```python
from build123d import *

# Parameters (mm, degrees)
SKETCH1_W           = 369
SKETCH1_H           = 81
BOSS_EXTRUDE1_DEPTH = 10
SKETCH2_W           = 23
SKETCH2_H           = 162
BOSS_EXTRUDE2_DEPTH = 38
SKETCH3_R           = 3.3
CUT_EXTRUDE1_DEPTH  = 13
SKETCH4_R           = 2.5
CUT_EXTRUDE2_DEPTH  = 163
SKETCH5_R           = 1.65
CUT_EXTRUDE3_DEPTH  = 24
CUT_EXTRUDE4_DEPTH  = 13


with BuildPart() as part:
    # Sketch1 → Boss-Extrude1 (new body)
    with BuildSketch(Plane.XY):
        with Locations((184.5, 40.5)):
            Rectangle(SKETCH1_W, SKETCH1_H)
    extrude(amount=BOSS_EXTRUDE1_DEPTH)

    # Sketch2 → Boss-Extrude2 (add)
    with BuildSketch(Plane(origin=(369, 0, 0), x_dir=(0, 0, -1), z_dir=(1, 0, 0))):
        with Locations((-11.5, 0)):
            Rectangle(SKETCH2_W, SKETCH2_H)
    extrude(amount=BOSS_EXTRUDE2_DEPTH)

    # Sketch3 → Cut-Extrude1 (cut)
    with BuildSketch(Plane(origin=(0, 0, 0), x_dir=(-1, 0, 0), z_dir=(0, 0, -1))):
        with Locations((-10, 71)):
            Circle(SKETCH3_R)
        with Locations((-10, 10)):
            Circle(SKETCH3_R)
        with Locations((-40, 10)):
            Circle(SKETCH3_R)
        with Locations((-40, 71)):
            Circle(SKETCH3_R)
    extrude(amount=-CUT_EXTRUDE1_DEPTH, mode=Mode.SUBTRACT)

    # Sketch4 → Cut-Extrude2 (cut, through all)
    with BuildSketch(Plane(origin=(0, 81, 0), x_dir=(1, 0, 0), z_dir=(0, 1, 0))):
        with Locations((388, -11.5)):
            Circle(SKETCH4_R)
    extrude(amount=-CUT_EXTRUDE2_DEPTH, mode=Mode.SUBTRACT)

    # Sketch5 → Cut-Extrude3 (cut, through all)
    with BuildSketch(Plane(origin=(0, 0, 0), x_dir=(-1, 0, 0), z_dir=(0, 0, -1))):
        with Locations((-378, -78)):
            Circle(SKETCH5_R)
        with Locations((-378, 78)):
            Circle(SKETCH5_R)
    extrude(amount=-CUT_EXTRUDE3_DEPTH, mode=Mode.SUBTRACT)

    # Sketch6 → Cut-Extrude4 (cut)
    with BuildSketch(Plane(origin=(0, 0, 0), x_dir=(-1, 0, 0), z_dir=(0, 0, -1))):
        with BuildLine():
            Line((-382, -78), (-382, -81))
            Line((-382, -81), (-374, -81))
            Line((-374, -81), (-374, -78))
            ThreePointArc((-374, -78), (-378, -74), (-382, -78))
        make_face()
        with BuildLine():
            Line((-374, 78), (-374, 81))
            Line((-374, 81), (-382, 81))
            Line((-382, 81), (-382, 78))
            ThreePointArc((-382, 78), (-378, 74), (-374, 78))
        make_face()
    extrude(amount=-CUT_EXTRUDE4_DEPTH, mode=Mode.SUBTRACT)


solid = part.part
```
Input: part model. Units: mm. Frame: model coordinates. A direction names the side the tool comes from. Round coordinates to 2 decimals unless told otherwise and drop trailing zeros. Write each loop counter-clockwise with the first axis right and the second up, starting at its lowest first coordinate (ties: lowest second). Pieces come first, ordered by that corner, then holes. Notation, with made-up numbers: (44.5, 65) - (90.5, 65) arc R28 cw to (90.5, 84) - close; hole circle Ø10 at (45, 5). An arc over 180 degrees is marked (long way). Write item = value, one per line.
(1) Pull-direction query (X, two-part tool) for faces 5 (the cylindrical face through (12.619, 7.992, 4.93)), 6 (the flat face through (388, -1, 23)), 7 (the flat face through (380, -77, 13)), 8 (the flat face through (0, 40, 5)); classes: +X half, -X half, draft (parallel to the pull), parting line (faces both ways), or undercut.
Geometry check:
face_5 = undercut
face_6 = draft
face_7 = undercut
face_8 = -X half
(2) Section query B-B on x = 167. Output: boundary loops of the cut face in (y, z), then the cut area to 3 significant figures.
Geometry check:
outline = (0, 0) - (81, 0) - (81, 10) - (0, 10) - close
area = 810 mm^2
(3) Access query for faces 1 (the flat face through (182, 0, 5)), 2 (the flat face through (376, 78, 13)), 3 (the cylindrical face through (378, -74, 6)), 4 (the flat face through (182, 41, 10)). Directions: +Z, -Z, +X, -X, +Y, -Y. A direction counts if a zero-diameter tool reaches every point of the face in a straight line with its end or side. Return the directions, or none.
Geometry check:
face_1 = +Z, -Z, -X, -Y
face_2 = -Z, +Y
face_3 = -Z, -Y
face_4 = +Z, -X, +Y, -Y
(4) Material intervals for probe 1 along Y at (x, z) = (10, 3); probe 2 along Y at (x, z) = (378, 17); probe 3 along X at (y, z) = (10.5, 18.75), sorted ascending.
Geometry check:
probe_1 = 0 to 6.7, 13.3 to 67.7, 74.3 to 81
probe_2 = -81 to -79.65, -76.35 to 76.35, 79.65 to 81
probe_3 = 369 to 407
(5) Section query A-A on y = 38.5. Output: boundary loops of the cut face in (x, z), then the cut area to 3 significant figures.
Geometry check:
outline = (0, 0) - (407, 0) - (407, 23) - (369, 23) - (369, 10) - (0, 10) - close; hole circle Ø5 at (388, 11.5)
area = 4,540 mm^2
(6) Contact query for flat-ended pins moving along their axis: pin 1 Ø6 at (y, z) = (-40, 2.5) entering from -X; pin 2 Ø2 at (x, y) = (376.5, -76.5) entering from -Z; pin 3 Ø3 at (x, y) = (54.5, 14) entering from +Z. Output: stop coordinate, or through.
Geometry check:
pin_1 = 369
pin_2 = 13
pin_3 = 10
